```python
from build123d import *

# Parameters (mm, degrees)
EXTRUDE_1_DEPTH     = 1
SKETCH_2_R          = 2.930453947
EXTRUDE_2_DEPTH     = 0.01
SKETCH_3_W          = 3.813800337
SKETCH_3_H          = 2.421486406
EXTRUDE_3_DEPTH     = 4
SKETCH_4_W          = 0.5
SKETCH_4_H          = 4
CUT_EXTRUDE_1_DEPTH = 0.3
SKETCH_5_W          = 0.5
SKETCH_5_H          = 4
CUT_EXTRUDE_2_DEPTH = 0.5
CHAMFER_1_SIZE      = 0.3
SKETCH_6_R          = 0.3
EXTRUDE_4_DEPTH     = 4
CUT_EXTRUDE_3_DEPTH = 2


with BuildPart() as part:
    # 草图1 → 凸台-拉伸1 (new body)
    with BuildSketch(Plane(origin=(0, 0, 0), x_dir=(1, 0, 0), z_dir=(0, 1, 0))):
        with BuildLine():
            Line((-8.818862275, 3.5), (-3.018862275, 3.5))
            ThreePointArc((-3.018862275, 3.5), (0.481137725, 0), (-3.018862275, -3.5))
            Line((-3.018862275, -3.5), (-8.818862275, -3.5))
            ThreePointArc((-8.818862275, -3.5), (-12.318862275, 0), (-8.818862275, 3.5))
        make_face()
    extrude(amount=EXTRUDE_1_DEPTH)

    # 草图2 → 凸台-拉伸2 (add)
    with BuildSketch(Plane(origin=(0, 1, 0), x_dir=(1, 0, 0), z_dir=(0, 1, 0))):
        with Locations(Location((-8.651499717, 0, 0), (0, 0, 90))):
            Circle(SKETCH_2_R)
    extrude(amount=EXTRUDE_2_DEPTH)

    # 草图3 → 凸台-拉伸3 (add)
    with BuildSketch(Plane(origin=(0, 0, 0), x_dir=(-1, 0, 0), z_dir=(0, -1, 0))):
        with Locations((3.751479011, 0)):
            Rectangle(SKETCH_3_W, SKETCH_3_H)
    extrude(amount=EXTRUDE_3_DEPTH)

    # 草图4 → 切除-拉伸1 (cut)
    with BuildSketch(Plane(origin=(0, 0, -1.210743203), x_dir=(-1, 0, 0), z_dir=(0, 0, -1))):
        with Locations((3.751479011, -2)):
            Rectangle(SKETCH_4_W, SKETCH_4_H)
    extrude(amount=-CUT_EXTRUDE_1_DEPTH, mode=Mode.SUBTRACT)

    # 草图5 → 切除-拉伸2 (cut)
    with BuildSketch(Plane.XY.offset(1.210743203)):
        with Locations((-3.751479011, -2)):
            Rectangle(SKETCH_5_W, SKETCH_5_H)
    extrude(amount=-CUT_EXTRUDE_2_DEPTH, mode=Mode.SUBTRACT)

    # 倒角1
    chamfer_1_edges = [part.edges().sort_by_distance(p)[0] for p in [
        (-5.658379179, -2, 1.210743203),
        (-5.658379179, -2, -1.210743203),
        (-1.844578842, -2, -1.210743203),
        (-1.844578842, -2, 1.210743203),
        (-4.001479011, -2, -1.210743203),
        (-3.501479011, -2, -1.210743203),
        (-3.501479011, -2, 1.210743203),
        (-4.001479011, -2, 1.210743203),
    ]]
    chamfer(chamfer_1_edges, length=CHAMFER_1_SIZE - 0.0001)  # a hair under: the kernel refuses the full size

    # 草图6 → 凸台-拉伸4 (add)
    with BuildSketch(Plane(origin=(0, -4, 0), x_dir=(-1, 0, 0), z_dir=(0, -1, 0))):
        with Locations(Location((2.673028926, 0, 0), (0, 0, 90))):
            Circle(SKETCH_6_R)
    extrude(amount=EXTRUDE_4_DEPTH)

    # 草图7 → 切除-拉伸3 (cut, symmetric)
    with BuildSketch(Plane.XY):
        Polygon((-2.973028926, -8), (-2.373028926, -6.485168842), (-2.373028926, -8), align=None)
    extrude(amount=CUT_EXTRUDE_3_DEPTH, both=True, mode=Mode.SUBTRACT)


solid = part.part
```
For this review, take the finished solid that the model builds, in its own axes (mm). A direction names the side the tool comes from. Round coordinates to 2 decimals unless told otherwise and drop trailing zeros. Loops run counter-clockwise (first coordinate to the right, second up) from the corner with the lowest first, then second, coordinate; pieces in that order, holes last.
Q1. Add section B-B on x = -4.75. Write out the cut boundary in (y, z), plus the area to 3 significant figures.
Result sheet:
outline: (-4, -1.21) - (0, -1.21) - (0, -3.5) - (1, -3.5) - (1, 3.5) - (0, 3.5) - (0, 1.21) - (-4, 1.21) - close
area: 16.7 mm2
Q2. Machinability: for faces 1 (the face through (-3, -2, -1.211)), 2 (the face through (-3, -2, 1.211)), 3 (the face through (-5.658, -2, 0)), 4 (the face through (-1.845, -2, 0)), which of the approach directions +Z, -Z, +X, -X, +Y, -Y give a long, thin tool a straight path to every point of the face, cutting with its end or side? Answer none if there is none.
Result sheet:
face 1: -Z, +X, -X, -Y
face 2: +Z, +X, -X, -Y
face 3: +Z, -Z, -X, -Y
face 4: +Z, -Z, +X, -Y
Q3. Insertion check: pin 1 Ø4 at (x, y) = (-3.5, -1) entering from +Z; pin 2 Ø0.8 at (x, y) = (-2.5, -1.5) entering from +Z; pin 3 Ø2 at (x, z) = (-3, 2.5) entering from +Y; pin 4 Ø1 at (x, z) = (-1.5, 0.5) entering from -Y. Each pin has a flat end and moves straight along its axis. Give the tip position at first contact, or say it passes through.
Result sheet:
pin 1: stops at z = 3.5
pin 2: stops at z = 1.21
pin 3: stops at y = 1
pin 4: stops at y = -4
Q4. To check wall thickness, follow line 1 along X through (y, z) = (-2, 0.75); line 2 along Y through (x, z) = (-3.5, 1); line 3 along X through (y, z) = (-2, 0). State the ranges of each line that lie inside material, in increasing order.
Result sheet:
line 1: x = -5.66 to -4, -3.5 to -1.84
line 2: y = 0 to 1
line 3: x = -5.66 to -1.84
